Answer from the drawing. Dimensions are ordinates in mm from the lowest x, y and z of the part. Give positions to 0.01 mm unless a question says otherwise; leave off trailing zeros. Order: outer loops, then holes, each group sorted by start corner. A loop starts at its lowest first (then second) coordinate and runs counter-clockwise, first axis right, second up. Notation, with made-up numbers: (52, 29.25) - (66, 29.25) arc R18 ccw to (66, 52.25) - close; hole circle Ø6 at (74, 72). An arc over 180 degrees is marked (long way). Answer in a Markdown table with one row per item.
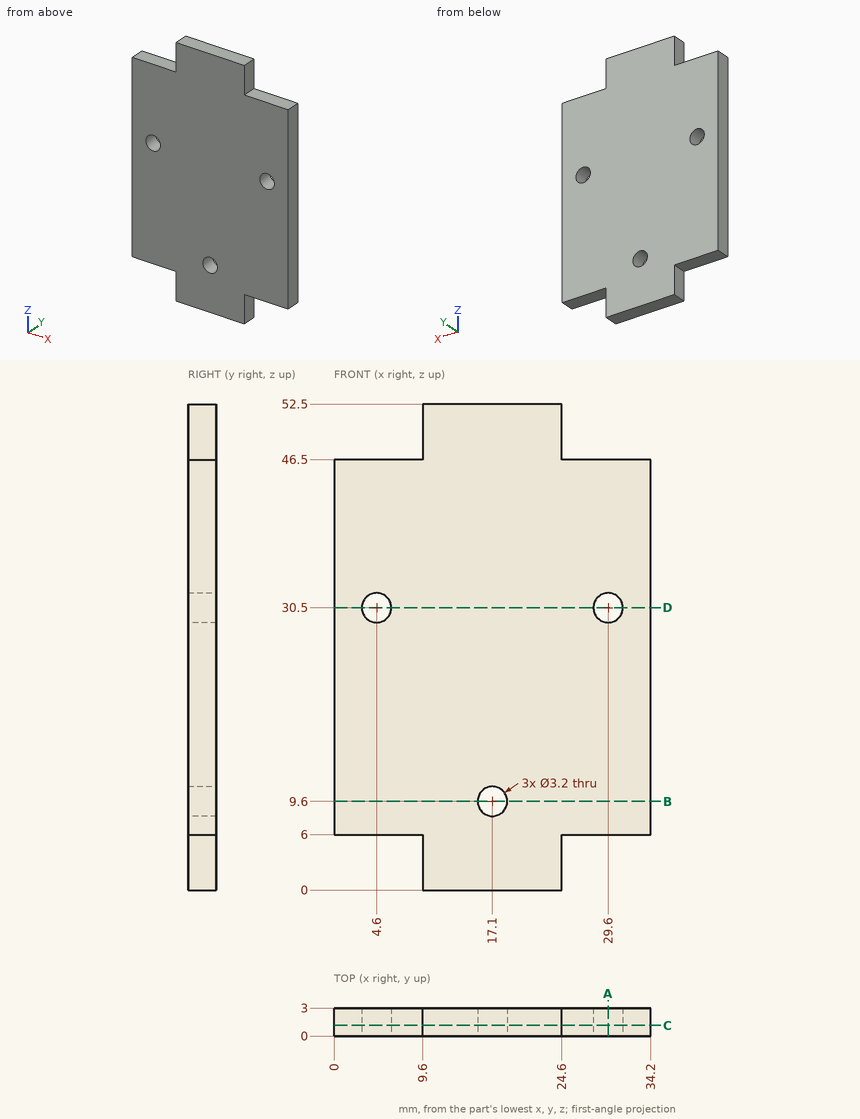
Item 1: Find section B-B on z = 9.6. Write down the section's boundary in (x, y).
Answer block:
| item | result |
|---|---|
| outline | (0, 0) - (15.5, 0) - (15.5, 3) - (0, 3) - close; (18.7, 0) - (34.2, 0) - (34.2, 3) - (18.7, 3) - close |
Item 2: Find section D-D on z = 30.5. Write down the section's boundary in (x, y).
Answer block:
| item | result |
|---|---|
| outline | (0, 0) - (3, 0) - (3, 3) - (0, 3) - close; (6.2, 0) - (28, 0) - (28, 3) - (6.2, 3) - close; (31.2, 0) - (34.2, 0) - (34.2, 3) - (31.2, 3) - close |
Item 3: Each of these flat-tipped pins is pushed along its axis until it touches: P1, Ø1.5, axis at y = 1, z = 50, coming from the -X side; P2, Ø0.9, axis at y = 1, z = 50, coming from the +X side; P3, Ø3, axis at x = 17.1, z = 9.6, coming from the +Y side; P4, Ø0.9, axis at x = 29.5, y = 1, coming from the +Z side. Where does it stop, or does it pass through?
Answer block:
| item | result |
|---|---|
| P1 | x = 9.6 |
| P2 | x = 24.6 |
| P3 | through |
| P4 | z = 46.5 |
Item 4: Consider line 1 (X direction, y = 0.9, z = 30.5); line 2 (Z direction, x = 17.1, y = 1.3); line 3 (Z direction, x = 29.6, y = 1.05). Determine where each line is inside the solid, lowest interval first.
Answer block:
| item | result |
|---|---|
| line 1 | 0 to 3, 6.2 to 28, 31.2 to 34.2 |
| line 2 | 0 to 8, 11.2 to 52.5 |
| line 3 | 6 to 28.9, 32.1 to 46.5 |
Item 5: Find section C-C on y = 1.15. Write down the section's boundary in (x, z).
Answer block:
| item | result |
|---|---|
| outline | (0, 6) - (9.6, 6) - (9.6, 0) - (24.6, 0) - (24.6, 6) - (34.2, 6) - (34.2, 46.5) - (24.6, 46.5) - (24.6, 52.5) - (9.6, 52.5) - (9.6, 46.5) - (0, 46.5) - close; hole circle Ø3.2 at (4.6, 30.5); hole circle Ø3.2 at (17.1, 9.6); hole circle Ø3.2 at (29.6, 30.5) |
Item 6: Find section A-A on x = 29.6. Write down the section's boundary in (y, z).
Answer block:
| item | result |
|---|---|
| outline | (0, 6) - (3, 6) - (3, 28.9) - (0, 28.9) - close; (0, 32.1) - (3, 32.1) - (3, 46.5) - (0, 46.5) - close |
